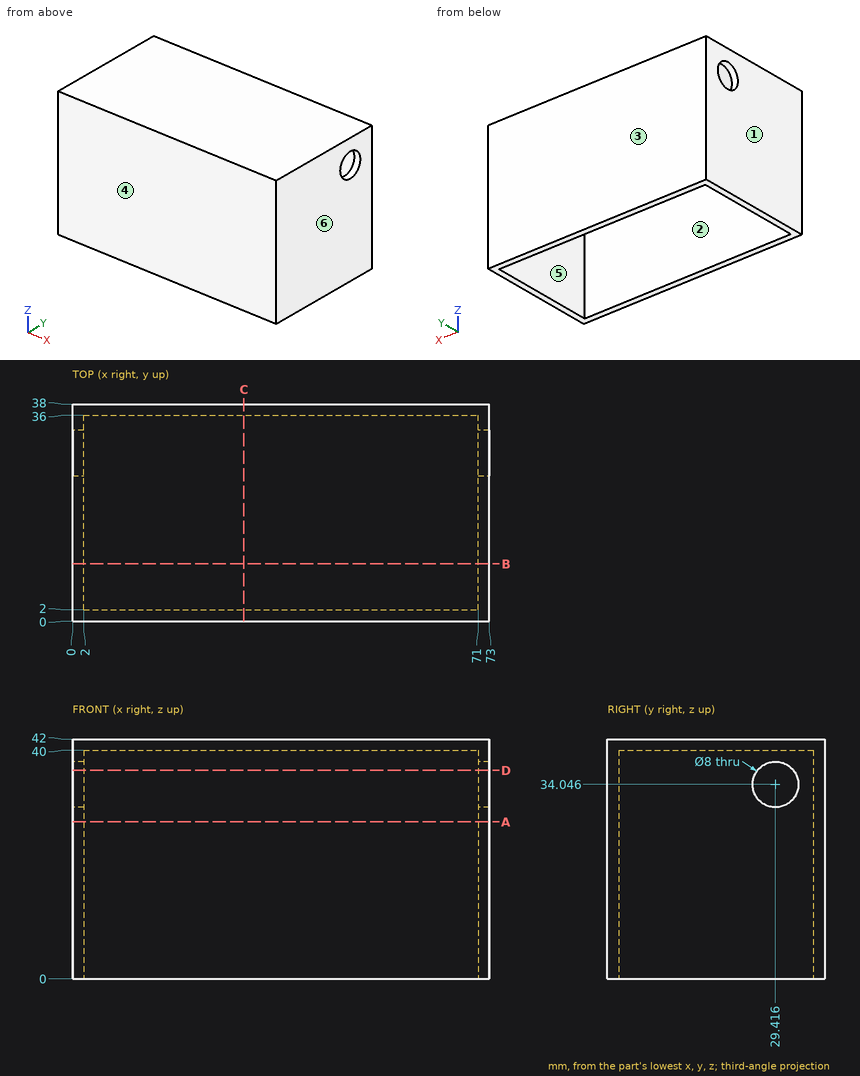
Job drawing, mm, ordinate dimensions from the low corner. One solid piece. A direction names the side the tool comes from. Coordinates: 2 decimals unless noted, no trailing zeros. Loops run counter-clockwise (first coordinate to the right, second up) from the corner with the lowest first, then second, coordinate; pieces in that order, holes last. Notation, with made-up numbers: (45, -7.75) - (95, -7.75) arc R16 cw to (95, 13.25) - close; hole circle Ø7 at (-9.5, 78). An arc over 180 degrees is marked (long way). Write item = value, one per line. Start each with the question number.
Q1. Cut at D-D, the plane z = 36.5. List the corners of the cut face in (x, y) (3 decimals), then the cut area to 3 significant figures.
Q2. Flat gauge pins, fed straight in: pin 1 Ø3 at (x, y) = (64, 7) entering from -Z; pin 2 Ø6 at (y, z) = (19, 10.5) entering from -X. Where does each tip first touch, or does it go through?
Q3. Cut at B-B, the plane y = 10. List the corners of the cut face in (x, z).
Q4. Cut at A-A, the plane z = 27.5. List the corners of the cut face in (x, y), then the cut area to 3 significant figures.
Q5. Pull direction Y, two halves, no side cores. Call the marked faces 3, 4, 5 and 6: pulls with the +Y half, pulls with the -Y half, needs draft (parallel to the pull), parting line crosses it, or undercut.
Q6. Drill centre lines: L1, parallel to Y at x = 53, z = 29; L2, parallel to X at y = 22.5, z = 8; L3, parallel to Z at x = 32, y = 21. Where is each one in solid material? Low to high.
Q7. Which spindle directions (+Z, -Z, +X, -X, +Y, -Y) get a long thin tool onto all of the face, cutting with end or side? Do the marked faces 1 and 2. Say none if no direction does.
Q8. Cut at C-C, the plane x = 30. List the corners of the cut face in (y, z), then the cut area to 3 significant figures.
Computed:
q1.outline = (0, 0) - (73, 0) - (73, 26.257) - (71, 26.257) - (71, 2) - (2, 2) - (2, 26.257) - (0, 26.257) - close; (0, 32.575) - (2, 32.575) - (2, 36) - (71, 36) - (71, 32.575) - (73, 32.575) - (73, 38) - (0, 38) - close
q1.area = 403 mm²
q2.pin_1 = 40
q2.pin_2 = 0
q3.outline = (0, 0) - (2, 0) - (2, 40) - (71, 40) - (71, 0) - (73, 0) - (73, 42) - (0, 42) - close
q4.outline = (0, 0) - (73, 0) - (73, 38) - (0, 38) - close; hole (2, 2) - (71, 2) - (71, 36) - (2, 36) - close
q4.area = 428 mm²
q5.face_3 = pulls with the +Y half
q5.face_4 = pulls with the -Y half
q5.face_5 = undercut
q5.face_6 = needs draft
q6.L1 = 0 to 2, 36 to 38
q6.L2 = 0 to 2, 71 to 73
q6.L3 = 40 to 42
q7.face_1 = +Z, -Z, -X, +Y, -Y
q7.face_2 = -Z
q8.outline = (0, 0) - (2, 0) - (2, 40) - (36, 40) - (36, 0) - (38, 0) - (38, 42) - (0, 42) - close
q8.area = 236 mm²
